Answer from the drawing. Dimensions are ordinates in mm from the lowest x, y and z of the part. A direction names the side the tool comes from. Coordinates: 2 decimals unless noted, no trailing zeros. Write each loop counter-clockwise with the first axis right and the second up, starting at its lowest first coordinate (ties: lowest second). Pieces come first, ordered by that corner, then holes. Notation, with made-up numbers: (6.5, 68) -> (26.5, 68) arc R30 ccw to (26.5, 107) -> close; hole circle Ø11 at (16.5, -15.75). An arc over 180 degrees is marked (long way). Answer as a JSON object with one key per item and string values. Group by question number.
(1) For a pull along Z with two mould halves and no side action, classify the marked faces 1, 2 and 3 as +Z half, -Z half, draft (parallel to the pull), parting line (faces both ways), or undercut.
(2) Find section B-B (z = 47). Give the vertices of the cut face in (x, y), then the cut area to 3 significant figures.
(3) Which of the six approach directions +Z, -Z, +X, -X, +Y, -Y give full straight-line access (tool end or side, diameter ignored) to the marked faces 4 and 5?
(4) Find section C-C (y = 13). Give the vertices of the cut face in (x, z).
(5) Straight lines are drawn through the part: L1, parallel to Z at x = 184, y = 19.25; L2, parallel to X at y = 14, z = 55.5; L3, parallel to Y at x = 90, z = 76. For each, find the intervals that lie inside material, in ascending order.
(6) Find section A-A (x = 186). Give the vertices of the cut face in (y, z), then the cut area to 3 significant figures.
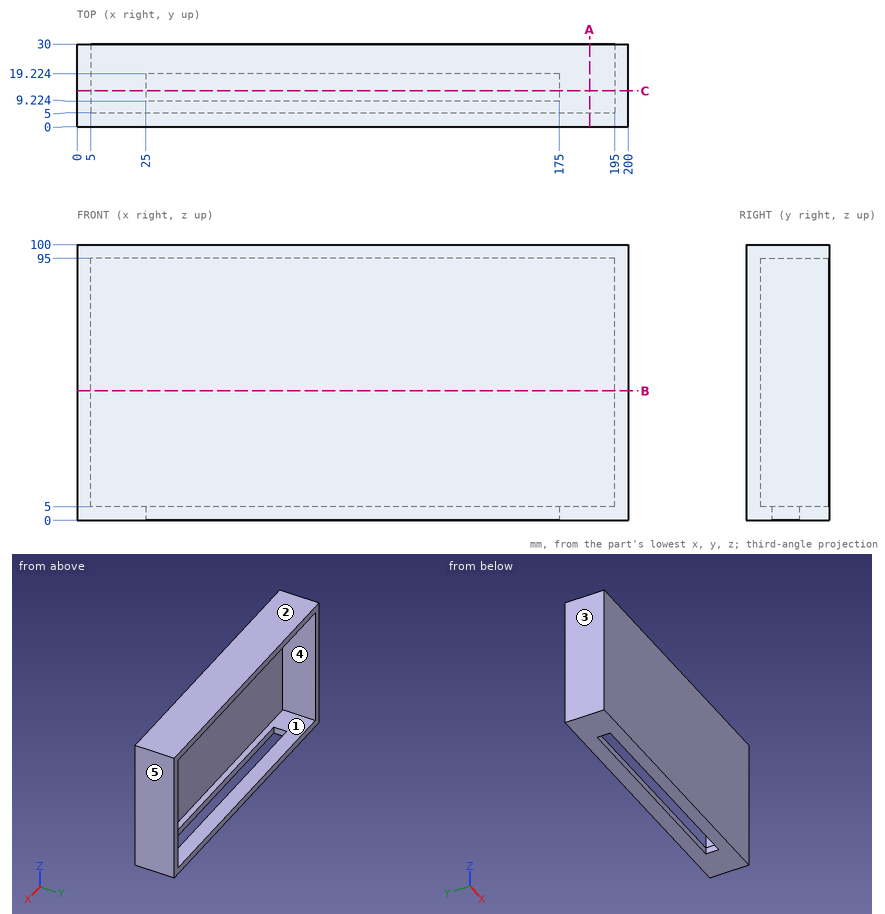
Results below:
{
 "1": {"face 1": "undercut", "face 2": "+Z half", "face 3": "draft"},
 "2": {"outline": "(0, 0) -> (200, 0) -> (200, 30) -> (195, 30) -> (195, 5) -> (5, 5) -> (5, 30) -> (0, 30) -> close", "area": "1,250 mm2"},
 "3": {"face 4": "+Y", "face 5": "+Z, -Z, +X, +Y, -Y"},
 "4": {"outline": "(0, 0) -> (25, 0) -> (25, 5) -> (5, 5) -> (5, 95) -> (195, 95) -> (195, 5) -> (175, 5) -> (175, 0) -> (200, 0) -> (200, 100) -> (0, 100) -> close"},
 "5": {"L1": "z = 0 to 5, 95 to 100", "L2": "x = 0 to 5, 195 to 200", "L3": "y = 0 to 5"},
 "6": {"outline": "(0, 0) -> (30, 0) -> (30, 5) -> (5, 5) -> (5, 95) -> (30, 95) -> (30, 100) -> (0, 100) -> close", "area": "750 mm2"}
}
